from build123d import *

# Parameters (mm, degrees)
F1_DEPTH = 75.565
F2_R     = 2.0955
F3_DEPTH = 13.97
F4_R     = 4
F5_DEPTH = 12.7
F6_R     = 4.2037
F7_DEPTH = 31.751


# Not quite as in the source:
# - a pattern or mirror of a feature is missing from the dataset's text; its kind, count and spacing are read off the source's solid


with BuildPart() as f1:
    # F0 (on Front) → F1 (new body, symmetric)
    with BuildSketch(Plane.XZ):
        Polygon((0, 31.75), (0, 0), (50.8, 0), (50.8, 10.16), (47.244, 10.16), (47.244, 18.542), (50.8, 18.542), (50.8, 19.304), (63.5, 19.304), (63.5, 18.542), (67.056, 18.542), (67.056, 10.16), (63.5, 10.16), (63.5, 0), (76.2, 0), (76.2, 31.75), (31.7754, 31.75), (31.7754, 25.146), (19.05, 25.146), (19.05, 31.75), align=None)
    extrude(amount=F1_DEPTH, both=True)

    # F2 (on face) → F3 (cut)
    with BuildSketch(Plane.XZ.offset(75.565)):
        with Locations((57.15, 25.9160771966)):
            Circle(F2_R)
    f3 = extrude(amount=-F3_DEPTH, mode=Mode.SUBTRACT)

    # F3_copies: F3 across plane
    add(f3.mirror(Plane.ZX), mode=Mode.SUBTRACT)

    # F4 (on face) → F5 (cut)
    with BuildSketch(Plane.YZ.offset(76.2)):
        with Locations((-50.673, 17.4752)):
            Circle(F4_R)
        with Locations((0.127, 17.4752)):
            Circle(F4_R)
        with Locations((50.927, 17.4752)):
            Circle(F4_R)
    extrude(amount=-F5_DEPTH, mode=Mode.SUBTRACT)

    # F6 (on face) → F7 (cut, through all)
    with BuildSketch(Plane.XY.offset(31.75)):
        with Locations((9.525, 57.785)):
            Circle(F6_R)
        with Locations((9.525, 26.035)):
            Circle(F6_R)
        with Locations((41.275, 26.035)):
            Circle(F6_R)
        with Locations((41.275, -43.815)):
            Circle(F6_R)
        with Locations((9.525, -43.815)):
            Circle(F6_R)
        with Locations((9.525, -66.675)):
            Circle(F6_R)
    extrude(amount=-F7_DEPTH, mode=Mode.SUBTRACT)


solid = f1.part
Build history of the part. All positions in model axes, mm. A direction names the side the tool comes from. Round coordinates to 2 decimals unless told otherwise and drop trailing zeros. Write each loop counter-clockwise with the first axis right and the second up, starting at its lowest first coordinate (ties: lowest second). Pieces come first, ordered by that corner, then holes. Notation, with made-up numbers: M 69,89.5 L 109,89.5 A12 ccw 109,96.5 Z; hole C -28,88.5 d1. An arc over 180 degrees is marked long. Answer as a JSON object with one key per item and string values. Group by question number.
(1) Cut at D-D (y = 59.5). Give the cut face in (x, z).
(2) Mould opens along Z. For faces 1 (the flat face through (76.2, -1, 12)), 2 (the flat face through (49, -1, 10.16)), 3 (the flat face through (10, -1, 31.75)), 4 (the cylindrical face through (69.94, -0.39, 21.44)) say: pulls with the +Z half, pulls with the -Z half, needs draft (parallel to the pull), parting line crosses it, or undercut.
(3) Cut at A-A (y = 37.5). Give the cut face in (x, z), and give its area (3 significant figures).
(4) Drill centre lines: L1, parallel to X at y = 58, z = 16; L2, parallel to X at y = 7.5, z = 15; L3, parallel to X at y = 5, z = 2. Where is each one in solid material? Low to high.
(5) Which spindle directions (+Z, -Z, +X, -X, +Y, -Y) get a long thin tool onto all of the face, cutting with end or side? Do faces 5 (the flat face through (19.05, -1, 28)), 6 (the cylindrical face through (56.877, 68.678, 27.994)), 7 (the flat face through (65, -65, 18.542)). Say none if no direction does.
(6) Cut at B-B (z = 15). Give the number of separate pieces and of enclosed holes in the cut face, and give its area (3 significant figures).
(7) Flat gauge pins, fed straight in: pin 1 (11 mm diameter, centred on y = 24, z = 6.5, fed in from -X); pin 2 (4 mm diameter, centred on x = 22.5, y = 17, fed in from +Z); pin 3 (1.7 mm diameter, centred on y = -51, z = 20, fed in from +X); pin 4 (1.3 mm diameter, centred on x = 57.5, z = 25, fed in from -Y) (3 decimals). Where does each tip first touch, or does it go through?
(8) Cut at C-C (x = 39). Give the cut face in (y, z) (3 decimals).
Responses:
{
 "1": {"outline": "M 0,0 L 5.69,0 L 5.69,31.75 L 0,31.75 Z; M 13.36,0 L 50.8,0 L 50.8,10.16 L 47.24,10.16 L 47.24,18.54 L 50.8,18.54 L 50.8,19.3 L 63.5,19.3 L 63.5,18.54 L 67.06,18.54 L 67.06,10.16 L 63.5,10.16 L 63.5,0 L 76.2,0 L 76.2,31.75 L 31.78,31.75 L 31.78,25.15 L 19.05,25.15 L 19.05,31.75 L 13.36,31.75 Z"},
 "2": {"face 1": "needs draft", "face 2": "undercut", "face 3": "pulls with the +Z half", "face 4": "undercut"},
 "3": {"outline": "M 0,0 L 50.8,0 L 50.8,10.16 L 47.24,10.16 L 47.24,18.54 L 50.8,18.54 L 50.8,19.3 L 63.5,19.3 L 63.5,18.54 L 67.06,18.54 L 67.06,10.16 L 63.5,10.16 L 63.5,0 L 76.2,0 L 76.2,31.75 L 31.78,31.75 L 31.78,25.15 L 19.05,25.15 L 19.05,31.75 L 0,31.75 Z", "area": "2,030 mm2"},
 "4": {"L1": "x = 0 to 5.33, 13.72 to 47.24, 67.06 to 76.2", "L2": "x = 0 to 47.24, 67.06 to 76.2", "L3": "x = 0 to 50.8, 63.5 to 76.2"},
 "5": {"face 5": "+Z, +Y, -Y", "face 6": "+Y", "face 7": "+Y, -Y"},
 "6": {"separate pieces": "5", "enclosed holes": "6", "area": "8,020 mm2"},
 "7": {"pin 1": "stops at x = 0", "pin 2": "stops at z = 25.15", "pin 3": "stops at x = 63.5", "pin 4": "stops at y = -61.595"},
 "8": {"outline": "M -75.565,0 L -47.35,0 L -47.35,31.75 L -75.565,31.75 Z; M -40.28,0 L 22.5,0 L 22.5,31.75 L -40.28,31.75 Z; M 29.57,0 L 75.565,0 L 75.565,31.75 L 29.57,31.75 Z"}
}
